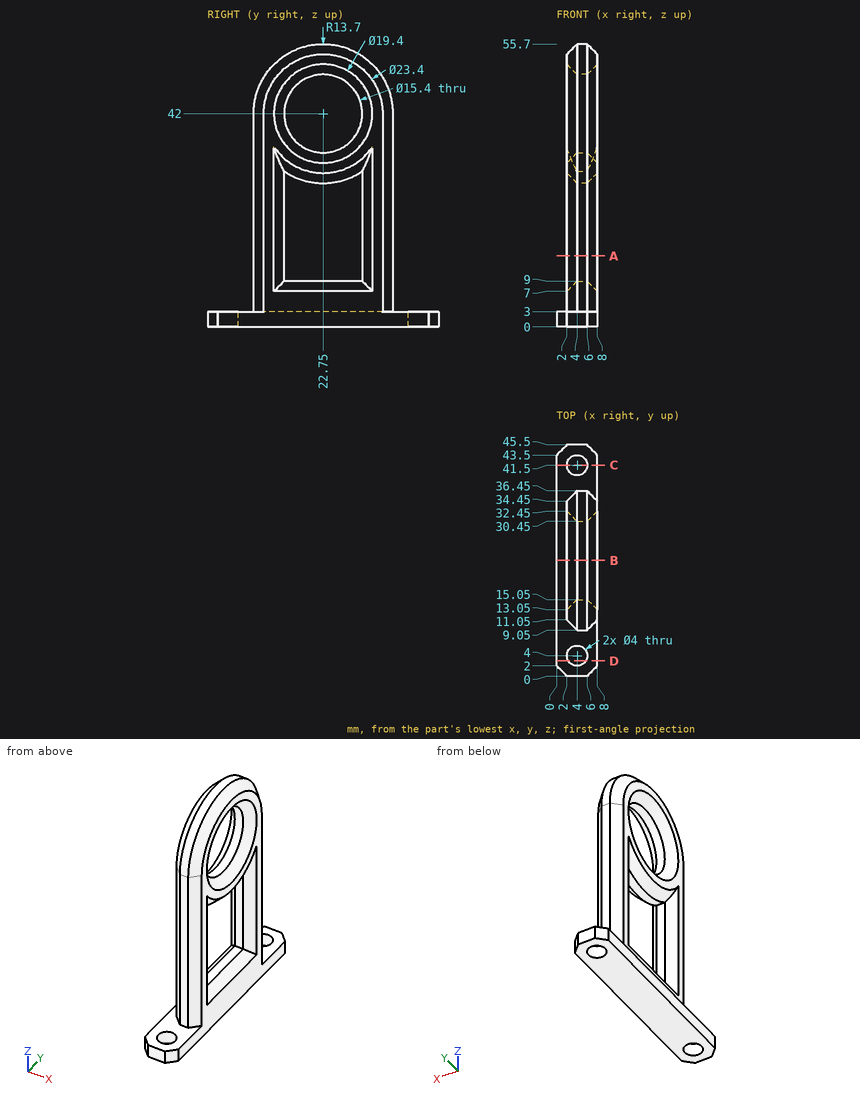
Input: dimensioned drawing with shaded views. Units: mm. Origin: part minimum x, y, z. Give positions to 0.01 mm unless a question says otherwise; leave off trailing zeros. Loops run counter-clockwise (first coordinate to the right, second up) from the corner with the lowest first, then second, coordinate; pieces in that order, holes last. Notation, with made-up numbers: (10.5, 82) -> (15.5, 82) arc R19 cw to (15.5, 96) -> close; hole circle Ø3 at (-35, -19.75). An arc over 180 degrees is marked (long way). Use a Markdown table: item, result. Add a question column.
1) Line query: line 1 along Y through (x, z) = (4, 1.05); line 2 along Z through (x, y) = (2.5, 25); line 3 along X through (y, z) = (4, 2.2). Output: solid intervals per line, ascending. Write a range as [from, to].
2) Section query C-C, the plane y = 41.5. Return the cut outline in (x, z), then the cut area to 3 significant figures.
3) Section query A-A, the plane z = 14. Return the cut outline in (x, y).
4) Section query D-D, the plane y = 3. Return the cut outline in (x, z).
5) First-contact query: pin 1 (5 mm diameter, centred on y = 5, z = 43, fed in from -X); pin 2 (4 mm diameter, centred on x = 6, y = 19.5, fed in from +Z); pin 3 (1.6 mm diameter, centred on x = 5, y = 21, fed in from +Z); pin 4 (2 mm diameter, centred on x = 5.5, z = 15, fed in from -Y). Flat tips, straight axial feed; report the tip coordinate or a pass-through.
6) Section query B-B, the plane y = 22.75. Return the cut outline in (x, z).
Numbers:
| question | item | result |
|---|---|---|
| 1 | line 1 | y = [0, 2], [6, 39.5], [43.5, 45.5] |
| 1 | line 2 | z = [0, 7.5], [30.01, 33.08], [50.92, 53.99] |
| 1 | line 3 | x = [0, 2], [6, 8] |
| 2 | outline | (0, 0) -> (2, 0) -> (2, 3) -> (0, 3) -> close; (6, 0) -> (8, 0) -> (8, 3) -> (6, 3) -> close |
| 2 | area | 12.0 mm2 |
| 3 | outline | (2, 11.05) -> (4, 9.05) -> (6, 9.05) -> (8, 11.05) -> (8, 13.05) -> (6, 15.05) -> (4, 15.05) -> (2, 13.05) -> close; (2, 32.45) -> (4, 30.45) -> (6, 30.45) -> (8, 32.45) -> (8, 34.45) -> (6, 36.45) -> (4, 36.45) -> (2, 34.45) -> close |
| 4 | outline | (0, 0) -> (2.27, 0) -> (2.27, 3) -> (0, 3) -> close; (5.73, 0) -> (8, 0) -> (8, 3) -> (5.73, 3) -> close |
| 5 | pin 1 | passes through |
| 5 | pin 2 | stops at z = 55.64 |
| 5 | pin 3 | stops at z = 55.67 |
| 5 | pin 4 | stops at y = 9.05 |
| 6 | outline | (0, 0) -> (8, 0) -> (8, 7) -> (6, 9) -> (4, 9) -> (2, 7) -> (2, 3) -> (0, 3) -> close; (2, 30.3) -> (4, 28.3) -> (6, 28.3) -> (8, 30.3) -> (8, 32.3) -> (6, 34.3) -> (4, 34.3) -> (2, 32.3) -> close; (2, 51.7) -> (4, 49.7) -> (6, 49.7) -> (8, 51.7) -> (8, 53.7) -> (6, 55.7) -> (4, 55.7) -> (2, 53.7) -> close |
